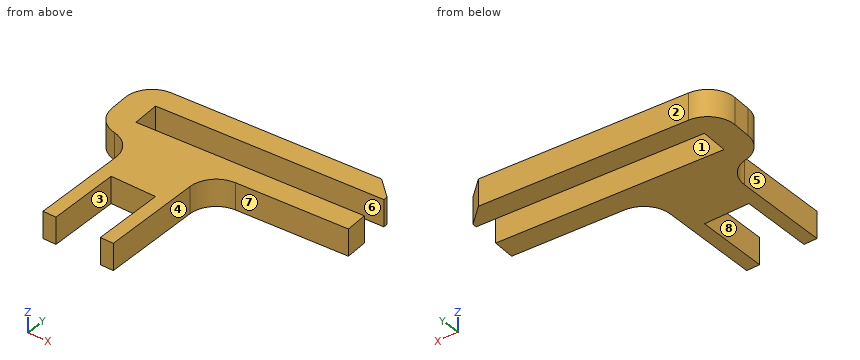
Autodesk Inventor part; units mm, degrees
ref_plane "YZ Plane" through (0, 0, 0) normal (1, 0, 0) x (0, 1, 0)
ref_plane "XZ Plane" through (0, 0, 0) normal (0, 1, 0) x (-1, 0, 0)
ref_plane "XY Plane" through (0, 0, 0) normal (0, 0, 1) x (1, 0, 0)
sketch "Sketch1" plane through (0, 0, 0) normal (0, 0, 1) x (1, 0, 0)
  line L0 (-4, -7) -> (4, -7)
  line L1 (4, -7) -> (4, 7)
  line L2 (4, 7) -> (-4, 7)
  line L3 (-4, 7) -> (-4, -7)
  line L4 (-4, -7) -> (4, 7) construction
  line L5 (4, -7) -> (-4, 7) construction
  line L6 (19.1902, 7.7382) -> (18.7715, 15.7272)
  line L7 (18.7715, 15.7272) -> (-9.1902, 14.2618)
  line L8 (-9.1902, 14.2618) -> (-8.7715, 6.2728)
  line L9 (-8.7715, 6.2728) -> (19.1902, 7.7382)
  line L10 (19.1902, 7.7382) -> (-9.1902, 14.2618) construction
  line L11 (18.7715, 15.7272) -> (-8.7715, 6.2728) construction
  line L12 (19.0606, 10.2098) -> (18.901, 13.2556)
  line L13 (18.901, 13.2556) -> (-6.0647, 11.9472)
  line L14 (-6.0647, 11.9472) -> (-5.9051, 8.9014)
  line L15 (-5.9051, 8.9014) -> (19.0606, 10.2098)
  line L16 (-8.9808, 10.2673) -> (18.9808, 11.7327)
  line L17 (-2.525, -7) -> (2.525, -7)
  line L18 (2.525, -7) -> (2.525, 1)
  line L19 (2.525, 1) -> (-2.525, 1)
  line L20 (-2.525, 1) -> (-2.525, -7)
  point P0 (0, 0)
  point P1 (0, 0)
  point P2 (5, 11)
  point P3 (5, 11)
  point P4 (5, 11)
  point P5 (0, 1)
  point P6 (0, -7)
  point P7 (-4, 6.5228)
  point P8 (4, 6.9421)
  point P9 (19.0606, 10.2098)
  point P10 (18.901, 13.2556)
  dimension "d19" = 8
  dimension "d20" = 14
  dimension "d21" = 5
  dimension "d22" = 3
  dimension "d23" = 4
  dimension "d24" = 8
  dimension "d25" = 28
  dimension "d27" = 3.05
  dimension "d29" = 25
  dimension "d30" = 5.05
  dimension "d31" = 8
extrude "Plate1" add sketch "Sketch1" along normal blind 3 contours L3 L9 L1 L0 L18 L19 L20 | L9 L8 L16 L14 L15 L6 L1 L2 L3 | L3 L2 L1 L9 | L8 L7 L6 L13 L14 L16
chamfer "Corner Chamfer1" distance 2 angle 45 1 edges at (18.7715, 15.7272, 1.5)
fillet "Corner Round2" radius 3 4 edges at (4, 6.9421, 1.5) (-8.7715, 6.2728, 1.5) (-4, 6.5228, 1.5) (-9.1902, 14.2618, 1.5)
equation "\"d14\" = Thickness"
equation "\"BendRadius\" = Thickness"
equation "\"BendReliefWidth\" = Thickness"
equation "\"BendReliefDepth\" = 0.5 * Thickness"
equation "\"CornerReliefSize\" = 4 * Thickness"
equation "\"MinimumRemnant\" = 2 * Thickness"
equation "\"TransitionRadius\" = BendRadius"
equation "\"JacobiRadiusSize\" = BendRadius"
equation "\"GapSize\" = Thickness"
properties part number "Path Plate Connector"
The model under review builds one solid part; all positions refer to its coordinate system, in mm. Face numbers are marked on the shaded views. A direction names the side the tool comes from. Give positions to 0.01 mm unless a question says otherwise; leave off trailing zeros. Order: outer loops, then holes, each group sorted by start corner. A loop starts at its lowest first (then second) coordinate and runs counter-clockwise, first axis right, second up. Notation, with made-up numbers: (-4, -35.5) -> (40, -35.5) arc R27 cw to (40, 1.5) -> close; hole circle Ø11 at (83.5, 18). An arc over 180 degrees is marked (long way). Write item = value, one per line. Start each with the question number.
(1) Take a section at D-D (y = 5). Write out the cut boundary in (x, z).
(2) For L1, parallel to X at y = -4.5, z = 0.7 (3 decimals); L2, parallel to X at y = 1.25, z = 2.2; L3, parallel to Y at x = 0.75, z = 2.2, list the stretches that pass through material, from the lowest coordinate up. Write a range as from..to.
(3) Tool access review of the marked faces 1, 2, 3, 4 and 5: name each direction out of +Z, -Z, +X, -X, +Y, -Y from which nothing blocks a thin tool from reaching the whole face with its end or side.
(4) Take a section at C-C (z = 0.5). Write out the cut boundary in (x, y) (3 decimals), plus the area to 3 significant figures.
(5) Take a section at B-B (y = -3.5). Write out the cut boundary in (x, z) (3 decimals), plus the area to 3 significant figures.
(6) Draft analysis for pull direction Y (two halves, no side actions). For the marked faces 6, 7 and 8, state which applies: +Y half, -Y half, draft (parallel to the pull), parting line (faces both ways), or undercut.
(7) Take a section at A-A (x = 1). Write out the cut boundary in (y, z).
(8) For pin 1 Ø1.5 at (x, y) = (6.5, -0.5) entering from +Z; pin 2 Ø1.5 at (y, z) = (-3, 2) entering from +X; pin 3 Ø0.9 at (y, z) = (-3, 2) entering from -X; pin 4 Ø1.5 at (x, z) = (-1, 1.5) entering from -Y, all flat-tipped, find the tip position at first contact; note any pin that passes through.
Returned:
q1.outline = (-4.39, 0) -> (4.14, 0) -> (4.14, 3) -> (-4.39, 3) -> close
q2.L1 = -4..-2.525, 2.525..4
q2.L2 = -4..4
q2.L3 = 1..9.25, 12.3..14.78
q3.face_1 = +Z, -Z
q3.face_2 = +Z, -Z, -X, +Y
q3.face_3 = +Z, -Z, -Y
q3.face_4 = +Z, -Z, +X, -Y
q3.face_5 = +Z, -Z, -X, -Y
q4.outline = (-9.033, 11.266) -> (-8.929, 9.269) arc R3 ccw to (-6.466, 6.474) arc R3 cw to (-4, 3.521) -> (-4, -7) -> (-2.525, -7) -> (-2.525, 1) -> (2.525, 1) -> (2.525, -7) -> (4, -7) -> (4, 4.095) arc R3 cw to (6.843, 7.091) -> (19.19, 7.738) -> (19.061, 10.21) -> (-5.905, 8.901) -> (-6.065, 11.947) -> (18.901, 13.256) -> (18.876, 13.73) -> (16.774, 15.623) -> (-6.194, 14.419) arc R3 ccw to start
q4.area = 215 mm²
q5.outline = (-4, 0) -> (-2.525, 0) -> (-2.525, 3) -> (-4, 3) -> close; (2.525, 0) -> (4, 0) -> (4, 3) -> (2.525, 3) -> close
q5.area = 8.85 mm²
q6.face_6 = undercut
q6.face_7 = -Y half
q6.face_8 = draft
q7.outline = (1, 0) -> (9.26, 0) -> (9.26, 3) -> (1, 3) -> close; (12.32, 0) -> (14.8, 0) -> (14.8, 3) -> (12.32, 3) -> close
q8.pin_1 = through
q8.pin_2 = 4
q8.pin_3 = -4
q8.pin_4 = 1
